Here's how the part is built. I have some questions about the finished solid (model axes, mm). A direction names the side the tool comes from. Round coordinates to 2 decimals unless told otherwise and drop trailing zeros. Write each loop counter-clockwise with the first axis right and the second up, starting at its lowest first coordinate (ties: lowest second). Pieces come first, ordered by that corner, then holes. Notation, with made-up numbers: (65, 18.25) -> (70, 18.25) arc R20 cw to (70, 29.25) -> close; hole circle Ø8 at (-25, -5). An arc over 180 degrees is marked (long way). Answer as CSV lines item,"result".
from build123d import *

# Parameters (mm, degrees)
SKETCH1_W            = 5.8
SKETCH1_H            = 5.2
BOSS_EXTRUDE1_DEPTH  = 8.5
BOSS_EXTRUDE2_DEPTH  = 0.5
SKETCH4_W            = 5.8
SKETCH4_H            = 1.1
BOSS_EXTRUDE3_DEPTH  = 1
BOSS_EXTRUDE6_START  = 0.5
SKETCH10_W           = 0.25
SKETCH10_H           = 0.2
BOSS_EXTRUDE6_DEPTH  = 2.2
BOSS_EXTRUDE7_START  = 0.07
SKETCH11_W           = 0.35
SKETCH11_H           = 0.291
BOSS_EXTRUDE7_DEPTH  = 3.72
LPATTERN3_COUNT      = 5
LPATTERN3_PITCH      = 0.635
LPATTERN3_COL_COUNT  = 5
LPATTERN3_COL_PITCH  = 0.635
LPATTERN4_COUNT      = 5
LPATTERN4_PITCH      = 0.64
LPATTERN4_COUNT_DIR2 = 5
LPATTERN4_PITCH_DIR2 = 0.64
SKETCH13_R           = 1.05
CUT_EXTRUDE1_DEPTH   = 0.1


with BuildPart() as part:
    # Sketch1 → Boss-Extrude1 (new body)
    with BuildSketch(Plane.XY):
        with Locations((2.9, 2.6)):
            Rectangle(SKETCH1_W, SKETCH1_H)
    extrude(amount=-BOSS_EXTRUDE1_DEPTH)

    # Sketch3 → Boss-Extrude2 (add)
    with BuildSketch(Plane.XY):
        with BuildLine():
            Line((1.588464453, 4.635827248), (4.211535547, 4.635827248))
            ThreePointArc((4.211535547, 4.635827248), (2.9, 0.178281999), (1.588464453, 4.635827248))
        make_face()
    extrude(amount=BOSS_EXTRUDE2_DEPTH)

    # Sketch4 → Boss-Extrude3 (add)
    with BuildSketch(Plane(origin=(0, 0, -8.5), x_dir=(-1, 0, 0), z_dir=(0, 0, -1))):
        with Locations((-2.9, 2.05)):
            Rectangle(SKETCH4_W, SKETCH4_H)
    extrude(amount=BOSS_EXTRUDE3_DEPTH)

    # Sketch10 → Boss-Extrude6 (add)
    with BuildSketch(Plane(origin=(0, 0, -8.5), x_dir=(-1, 0, 0), z_dir=(0, 0, -1)).offset(BOSS_EXTRUDE6_START)):
        with Locations((-2.9, 2.7)):
            Rectangle(SKETCH10_W, SKETCH10_H)
    boss_extrude6 = extrude(amount=BOSS_EXTRUDE6_DEPTH)

    # Sketch11 → Boss-Extrude7 (add)
    with BuildSketch(Plane(origin=(0, 0, -9.5), x_dir=(-1, 0, 0), z_dir=(0, 0, -1)).offset(BOSS_EXTRUDE7_START)):
        with Locations((-2.9, 2.5545)):
            Rectangle(SKETCH11_W, SKETCH11_H)
    boss_extrude7 = extrude(amount=BOSS_EXTRUDE7_DEPTH)

    # LPattern3: Boss-Extrude6 ×5
    with Locations(*[(-i * LPATTERN3_PITCH, 0, 0) for i in range(1, LPATTERN3_COUNT)]):
        add(boss_extrude6)

    # LPattern3 col: Boss-Extrude6 ×5
    with Locations(*[(i * LPATTERN3_COL_PITCH, 0, 0) for i in range(1, LPATTERN3_COL_COUNT)]):
        add(boss_extrude6)

    # LPattern4: Boss-Extrude7 5 × 5, 7 skipped
    with Locations(*[Vector(-1, 0, 0) * (i * LPATTERN4_PITCH) + Vector(1, 0, 0) * (j * LPATTERN4_PITCH_DIR2) for i in range(LPATTERN4_COUNT) for j in range(LPATTERN4_COUNT_DIR2) if (i, j) not in ((0, 0), (0, 1), (0, 2), (1, 2), (1, 3), (2, 3), (2, 4), (3, 4))]):
        add(boss_extrude7)

    # Sketch13 → Cut-Extrude1 (cut)
    with BuildSketch(Plane.XY.offset(0.5)):
        with Locations((2.9, 2.6)):
            Circle(SKETCH13_R)
    extrude(amount=-CUT_EXTRUDE1_DEPTH, mode=Mode.SUBTRACT)


solid = part.part
Item 1: Suppose I cut it at B-B, the plane y = 0.6. List the corners of the cut face in (x, z) for me, then the cut area to 3 significant figures.
Results found:
outline,"(0, -8.5) -> (5.8, -8.5) -> (5.8, 0) -> (4.27, 0) -> (4.27, 0.5) -> (1.53, 0.5) -> (1.53, 0) -> (0, 0) -> close"
area,"50.7 mm²"
Item 2: Suppose I cut it at A-A, the plane y = 3.1. List the corners of the cut face in (x, z) for me, then the cut area to 3 significant figures.
Results found:
outline,"(0, -8.5) -> (5.8, -8.5) -> (5.8, 0) -> (5.27, 0) -> (5.27, 0.5) -> (3.82, 0.5) -> (3.82, 0.4) -> (1.98, 0.4) -> (1.98, 0.5) -> (0.53, 0.5) -> (0.53, 0) -> (0, 0) -> close"
area,"51.5 mm²"
Item 3: Suppose I cut it at C-C, the plane y = 1.8. List the corners of the cut face in (x, z) for me.
Results found:
outline,"(0, -9.5) -> (5.8, -9.5) -> (5.8, 0) -> (5.19, 0) -> (5.19, 0.5) -> (3.58, 0.5) -> (3.58, 0.4) -> (2.22, 0.4) -> (2.22, 0.5) -> (0.61, 0.5) -> (0.61, 0) -> (0, 0) -> close"
Item 4: For faces 1 (the flat face through (3, 1, 0.5)), 2 (the cylindrical face through (2.99, 0.18, 0.25)), 3 (the flat face through (3, 1, -8.5)), 4 (the flat face through (3, 2, -9.5)), which set-ups out of +Z, -Z, +X, -X, +Y, -Y let a thin tool reach every point of the face, with its end or its side?
Results found:
face 1,"+Z, +X, -X, +Y, -Y"
face 2,"+Z"
face 3,"-Z, +X, -X, -Y"
face 4,"+X, -X, -Y"
Item 5: Will these pins go through, and if not, where does the flat tip stop? pin 1 (2.5 mm diameter, centred on x = 3.5, y = 2.5, fed in from +Z); pin 2 (0.9 mm diameter, centred on x = 3.5, y = 2, fed in from -Z); pin 3 (1 mm diameter, centred on x = 1, z = -9.5, fed in from -Y).
Results found:
pin 1,"stops at z = 0.5"
pin 2,"stops at z = -9.5"
pin 3,"stops at y = 1.5"
Item 6: I need wall thicknesses on L1, parallel to Z at x = 4.85, y = 0.7; L2, parallel to Z at x = 1.85, y = 3; L3, parallel to Y at x = 4.8, z = -8.75. Which ranges of each line are inside material? Lowest first, please.
Results found:
L1,"z = -8.5 to 0"
L2,"z = -8.5 to 0.5"
L3,"y = 1.5 to 2.6"
Item 7: If we mould it in two halves opening along Y, with no side actions, what happens to faces 5 (the flat face through (3, 5, 0)), 6 (the flat face through (3, 0, -4)), 7 (the flat face through (3, 3, 0.4))? For each: pulls with the +Y half, pulls with the -Y half, needs draft (parallel to the pull), parting line crosses it, or undercut.
Results found:
face 5,"needs draft"
face 6,"pulls with the -Y half"
face 7,"undercut"
